from build123d import *

# Parameters (mm, degrees)
BOSS_EXTRUDE1_DEPTH = 11.1125
HOLE1_D             = 7.1374
HOLE2_D             = 7.1374
FILLET1_R           = 0.381
FILLET2_R           = 3.175


with BuildPart() as part:
    # Sketch1 → Boss-Extrude1 (new, symmetric)
    with BuildSketch(Plane(origin=(0, 0, -11.1125), x_dir=(-1, 0, 0), z_dir=(0, 0, -1))):
        with BuildLine():
            Line((-25.4, 0), (0, 0))
            Line((0, 0), (0, 25.4))
            ThreePointArc((0, 25.4), (-3.376576302, 24.001376301), (-4.7752, 20.6248))
            Line((-4.7752, 20.6248), (-4.7752, 4.7752))
            Line((-4.7752, 4.7752), (-20.6248, 4.7752))
            ThreePointArc((-20.6248, 4.7752), (-24.001376302, 3.376576301), (-25.4, 0))
        make_face()
    extrude(amount=BOSS_EXTRUDE1_DEPTH, both=True)

    # Hole1 (through all)
    with Locations(Plane(origin=(0, 4.7752, 0), x_dir=(-1, 0, 0), z_dir=(0, 1, 0))):
        with Locations((-12.7, -11.1125)):
            Hole(HOLE1_D / 2)

    # Hole2 (through all)
    with Locations(Plane(origin=(4.7752, 0, 0), x_dir=(0, 0, -1), z_dir=(1, 0, 0))):
        with Locations((11.1125, 12.7)):
            Hole(HOLE2_D / 2)

    # Fillet1
    fillet1_edges = [part.edges().sort_by_distance(p)[0] for p in [
        (0, 0, -11.1125),
    ]]
    fillet(fillet1_edges, radius=FILLET1_R)

    # Fillet2
    fillet2_edges = [part.edges().sort_by_distance(p)[0] for p in [
        (4.7752, 4.7752, -11.1125),
    ]]
    fillet(fillet2_edges, radius=FILLET2_R)


solid = part.part
The model under review builds one solid part; all positions refer to its coordinate system, in mm. A direction names the side the tool comes from. Give positions to 0.01 mm unless a question says otherwise; leave off trailing zeros. Order: outer loops, then holes, each group sorted by start corner. A loop starts at its lowest first (then second) coordinate and runs counter-clockwise, first axis right, second up. Notation, with made-up numbers: (45.5, 79.5) -> (95.5, 79.5) arc R12 ccw to (95.5, 88.5) -> close; hole circle Ø8 at (-18, -26). An arc over 180 degrees is marked (long way). Write item = value, one per line. Start each with the question number.
(1) Take a section at C-C (z = -12). Write out the cut boundary in (x, y) (3 decimals), plus the area to 3 significant figures.
(2) Draft analysis for pull direction Z (two halves, no side actions). For faces 1 (the flat face through (0, 10, -14)), 2 (the flat face through (7, 4, -22.225)), 3 (the cylindrical face through (2.354, 12.857, -14.678)), state which applies: +Z half, -Z half, draft (parallel to the pull), parting line (faces both ways), or undercut.
(3) Take a section at A-A (x = 12.7). Write out the cut boundary in (y, z) (3 decimals), plus the area to 3 significant figures.
(4) For pin 1 Ø11.5 at (y, z) = (12.7, -11.11) entering from -X; pin 2 Ø8 at (x, z) = (19.5, -17) entering from +Y; pin 3 Ø12 at (x, z) = (7, -8) entering from +Y; pin 4 Ø6.5 at (y, z) = (11.5, -9) entering from +X, all flat-tipped, find the tip position at first contact; note any pin that passes through.
(5) Tool access review of faces 4 (the flat face through (16, 0, -9)), 5 (the flat face through (17, 4.775, -11)): name each direction out of +Z, -Z, +X, -X, +Y, -Y from which nothing blocks a thin tool from reaching the whole face with its end or side.
(6) Take a section at D-D (z = -3.5). Write out the cut boundary in (x, y) (3 decimals).
(7) For L1, parallel to X at y = 13.25, z = -17; L2, parallel to X at y = 4, z = -11, list the stretches that pass through material, from the lowest coordinate up. Write a range as from..to.
Returned:
q1.outline = (0, 0.381) arc R0.381 ccw to (0.381, 0) -> (9.243, 0) -> (9.243, 4.775) -> (7.95, 4.775) arc R3.175 cw to (4.775, 7.95) -> (4.775, 9.243) -> (0, 9.243) -> close; (0, 16.157) -> (4.775, 16.157) -> (4.775, 20.625) arc R4.775 ccw to (0, 25.4) -> close; (16.157, 0) -> (25.4, 0) arc R4.775 ccw to (20.625, 4.775) -> (16.157, 4.775) -> close
q1.area = 146 mm²
q2.face_1 = draft
q2.face_2 = -Z half
q2.face_3 = undercut
q3.outline = (0, -22.225) -> (4.775, -22.225) -> (4.775, -14.681) -> (0, -14.681) -> close; (0, -7.544) -> (4.775, -7.544) -> (4.775, 0) -> (0, 0) -> close
q3.area = 72.0 mm²
q4.pin_1 = 0
q4.pin_2 = 4.78
q4.pin_3 = 25.29
q4.pin_4 = 4.78
q5.face_4 = +Z, -Z, +X, -X, -Y
q5.face_5 = +Z, -Z, +X, +Y
q6.outline = (0, 0.381) arc R0.381 ccw to (0.381, 0) -> (25.4, 0) arc R4.775 ccw to (20.625, 4.775) -> (7.95, 4.775) arc R3.175 cw to (4.775, 7.95) -> (4.775, 20.625) arc R4.775 ccw to (0, 25.4) -> close
q7.L1 = 0..4.78
q7.L2 = 0..9.13, 16.27..23.23
